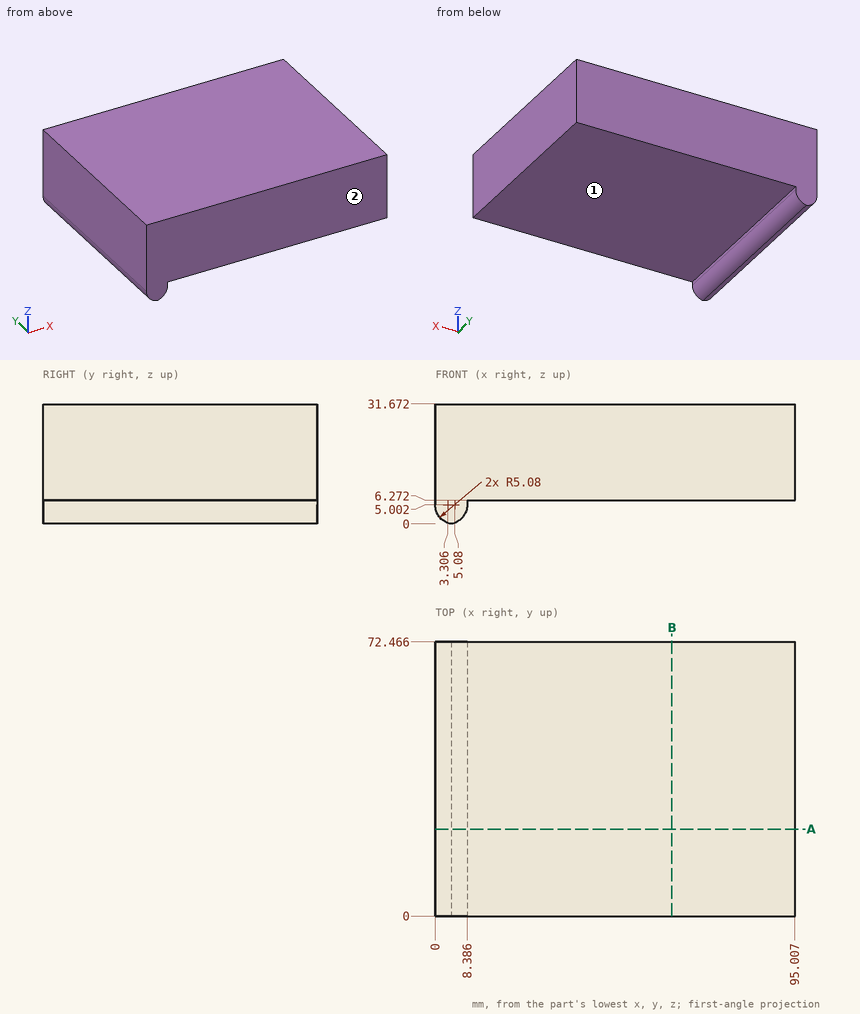
Input: dimensioned drawing with shaded views. Units: mm. Origin: part minimum x, y, z. A direction names the side the tool comes from. Coordinates: 2 decimals unless noted, no trailing zeros. Order: outer loops, then holes, each group sorted by start corner. A loop starts at its lowest first (then second) coordinate and runs counter-clockwise, first axis right, second up.
1. Cut plane A-A, the plane y = 23. Return loops of the section in (x, z).
Checked values:
outline: (0, 5) arc R5.08 ccw to (4.19, 0) arc R5.08 ccw to (8.39, 5) - (8.39, 6.27) - (95.01, 6.27) - (95.01, 31.67) - (0, 31.67) - close
2. Access query for the marked faces 1 and 2. Directions: +Z, -Z, +X, -X, +Y, -Y. A direction counts if a zero-diameter tool reaches every point of the face in a straight line with its end or side. Return the directions, or none.
Checked values:
face 1: -Z, +X, +Y, -Y
face 2: +Z, -Z, +X, -X, -Y
3. Cut plane B-B, the plane x = 62.5. Return loops of the section in (y, z).
Checked values:
outline: (0, 6.27) - (72.47, 6.27) - (72.47, 31.67) - (0, 31.67) - close
4. Contact query for a flat-ended pin moving along its axis: P1, Ø3, axis at x = 55.5, y = 15.5, coming from the -Z side. Output: stop coordinate, or through.
Checked values:
P1: stops at z = 6.27
5. Ray query, line 1 along X through (y, z) = (36, 6); line 2 along Z through (x, y) = (68, 67); line 3 along Z through (x, y) = (5, 43). Return the intervals inside material, ascending.
Checked values:
line 1: x = 0 to 8.39
line 2: z = 6.27 to 31.67
line 3: z = 0.21 to 31.67
